Part model, mm, in its own coordinate system. Face numbers are marked on the shaded views. A direction names the side the tool comes from. Give positions to 0.01 mm unless a question says otherwise; leave off trailing zeros. Loops run counter-clockwise (first coordinate to the right, second up) from the corner with the lowest first, then second, coordinate; pieces in that order, holes last. Notation, with made-up numbers: (71, 56) -> (118, 56) arc R31 cw to (118, 93) -> close; hole circle Ø7 at (85, 64). An arc over 180 degrees is marked (long way). One line per question, with ' | ' between items.
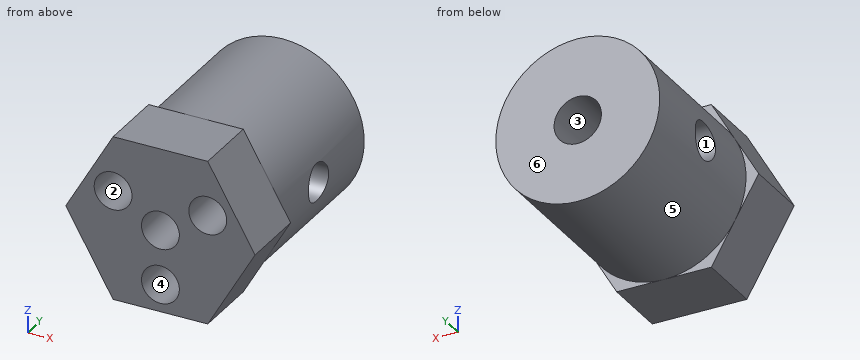
```python
from build123d import *

# Parameters (mm, degrees)
EXTRUDE_1_DEPTH          = 7
SKETCH_5_R               = 8.660254038
SKETCH_5_R_2             = 2.5
EXTRUDE_2_DEPTH          = 17
SKETCH_2_R               = 2
CUT_EXTRUDE_4_DEPTH      = 7
CUT_EXTRUDE_5_DEPTH      = 28.404379212
CUT_EXTRUDE_5_DEPTH_BACK = 28.404379212
SKETCH_6_R               = 2


with BuildPart() as part:
    # 草图1 → 凸台-拉伸1 (new body)
    with BuildSketch(Plane(origin=(0, 0, 0), x_dir=(1, 0, 0), z_dir=(0, 1, 0))):
        Polygon((10, 0), (5, 8.660254038), (-5, 8.660254038), (-10, 0), (-5, -8.660254038), (5, -8.660254038), align=None)
    extrude(amount=EXTRUDE_1_DEPTH)

    # 草图5 → 凸台-拉伸2 (add)
    with BuildSketch(Plane(origin=(0, 7, 0), x_dir=(1, 0, 0), z_dir=(0, 1, 0))):
        with Locations(Location((0, 0, 0), (0, 0, 270))):
            Circle(SKETCH_5_R)
        with Locations(Location((0, 0, 0), (0, 0, 270))):
            Circle(SKETCH_5_R_2, mode=Mode.SUBTRACT)
    extrude(amount=EXTRUDE_2_DEPTH)

    # 草图2 → 切除-拉伸4 (cut)
    with BuildSketch(Plane.XZ):
        with Locations(Location((0, 0, 0), (0, 0, 270))):
            Circle(SKETCH_2_R)
        with Locations(Location((-5, 2.886751346, 0), (0, 0, 270))):
            Circle(SKETCH_2_R)
        with Locations(Location((5, 2.886751346, 0), (0, 0, 270))):
            Circle(SKETCH_2_R)
        with Locations(Location((0, -5.773502692, 0), (0, 0, 270))):
            Circle(SKETCH_2_R)
    extrude(amount=-CUT_EXTRUDE_4_DEPTH, mode=Mode.SUBTRACT)

    # 草图6 → 切除-拉伸5 (cut, two sides: drawn at the far end of the back side and taken through both)
    with BuildSketch(Plane(origin=(0, 0, 0), x_dir=(0, 0, -1), z_dir=(1, 0, 0)).offset(-CUT_EXTRUDE_5_DEPTH_BACK)):
        with Locations((0, 15)):
            Circle(SKETCH_6_R)
    extrude(amount=CUT_EXTRUDE_5_DEPTH + CUT_EXTRUDE_5_DEPTH_BACK, mode=Mode.SUBTRACT)


solid = part.part
```
1) Saw through at B-B (y = 2.75). Give the cut face in (x, z), and give its area (3 significant figures).
Found:
outline: (-10, 0) -> (-5, -8.66) -> (5, -8.66) -> (10, 0) -> (5, 8.66) -> (-5, 8.66) -> close; hole circle Ø4 at (-5, 2.89); hole circle Ø4 at (0, -5.77); hole circle Ø4 at (0, 0); hole circle Ø4 at (5, 2.89) | area: 210 mm2
2) Saw through at D-D (z = -1). Give the cut face in (x, y), and give its area (3 significant figures).
Found:
outline: (-9.42, 0) -> (-1.73, 0) -> (-1.73, 7) -> (-2.29, 7) -> (-2.29, 13.27) -> (-8.6, 13.27) -> (-8.6, 7) -> (-9.42, 7) -> close; (-8.6, 16.73) -> (-2.29, 16.73) -> (-2.29, 24) -> (-8.6, 24) -> close; (1.73, 0) -> (9.42, 0) -> (9.42, 7) -> (8.6, 7) -> (8.6, 13.27) -> (2.29, 13.27) -> (2.29, 7) -> (1.73, 7) -> close; (2.29, 16.73) -> (8.6, 16.73) -> (8.6, 24) -> (2.29, 24) -> close | area: 279 mm2
3) Pull direction Z, two halves, no side cores. Call the marked faces 4, 5 and 6: pulls with the +Z half, pulls with the -Z half, needs draft (parallel to the pull), parting line crosses it, or undercut.
Found:
face 4: undercut | face 5: parting line crosses it | face 6: needs draft
4) Tool access for the marked faces 1, 2 and 3: list every direction of +Z, -Z, +X, -X, +Y, -Y with a clear straight run to the whole face (end or side of a thin tool).
Found:
face 1: +X, -X | face 2: -Y | face 3: +Y
5) Saw through at C-C (x = -3.75). Give the cut face in (y, z), and give its area (3 significant figures).
Found:
outline: (0, -8.66) -> (7, -8.66) -> (7, -7.81) -> (24, -7.81) -> (24, 7.81) -> (7, 7.81) -> (7, 8.66) -> (0, 8.66) -> (0, 4.45) -> (7, 4.45) -> (7, 1.33) -> (0, 1.33) -> close; hole circle Ø4 at (15, 0) | area: 352 mm2
6) Saw through at A-A (y = 15). Give the cut face in (x, z), and give its area (3 significant figures).
Found:
outline: (-8.43, -2) arc R8.66 ccw to (8.43, -2) -> (1.5, -2) arc R2.5 cw to (-1.5, -2) -> close; (-8.43, 2) -> (-1.5, 2) arc R2.5 cw to (1.5, 2) -> (8.43, 2) arc R8.66 ccw to start | area: 165 mm2
7) Drill centre lines: line 1 (X direction, y = 5.25, z = 1.75); line 2 (Z direction, x = -3.75, y = 15); line 3 (Z direction, x = -7.25, y = 13.75). Where is each one in solid material? Low to high.
Found:
line 1: -8.99 to -6.65, -3.35 to -0.97, 0.97 to 3.35, 6.65 to 8.99 | line 2: -7.81 to -2, 2 to 7.81 | line 3: -4.74 to -1.56, 1.56 to 4.74
8) Pin check, flat tips, straight feed: P1, Ø0.8, axis at x = -9.5, z = -1, coming from the +Y side; P2, Ø4.5, axis at x = -0.5, z = -5.5, coming from the -Y side; P3, Ø2.5, axis at x = 5, z = 2.89, coming from the -Y side; P4, Ø6, axis at y = 19, z = -1, coming from the -X side. Stop position of each tip, or through.
Found:
P1: y = 7 | P2: y = 0 | P3: y = 7 | P4: x = -8.66
